Autodesk Inventor part; units mm, degrees
ref_plane "YZ Plane" through (0, 0, 0) normal (1, 0, 0) x (0, 1, 0)
ref_plane "XZ Plane" through (0, 0, 0) normal (0, 1, 0) x (-1, 0, 0)
ref_plane "XY Plane" through (0, 0, 0) normal (0, 0, 1) x (1, 0, 0)
sketch "Sketch1" plane through (0, 0, 0) normal (0, 0, 1) x (1, 0, 0)
  arc A0 (0, 0) -> (0, -180) centre (45.304, -90) ccw
  line L0 (-55.4554, -90) -> (-45.4554, -90) construction
  line L1 (0, -180) -> (0, -170) construction
  line L2 (0, 0) -> (0, -10) construction
  line L3 (0, -180) -> (10, -180) construction
  line L4 (0, 0) -> (10, 0) construction
  arc A1 (10, 0) -> (10, -180) centre (55.304, -90) ccw
  line L5 (0, 0) -> (10, 0)
  line L6 (10, -180) -> (0, -180)
  dimension "d0" = 180
  dimension "d1" = 10
  dimension "d2" = 10
  dimension "d3" = 10
  dimension "d4" = 10
  dimension "d5" = 10
extrude "Extrusion1" add sketch "Sketch1" along normal blind 10
sketch "Sketch2" plane through (0, 0, 0) normal (0, 1, 0) x (1, 0, 0)
  line L0 (-55.4554, -10) -> (0, -10)
  line L1 (0, -10) -> (0, -15)
  line L2 (0, -15) -> (0, 5)
  line L3 (0, 5) -> (6, 5)
  line L4 (0, -15) -> (6, -15)
  line L5 (6, -15) -> (18, -10)
  line L6 (6, 5) -> (18, 0)
  line L7 (18, 0) -> (18, -10)
  point P0 (0, 0)
  dimension "d8" = 5
  dimension "d9" = 20
  dimension "d10" = 6
  dimension "d11" = 13
extrude "Extrusion2" add sketch "Sketch2" along normal blind 5
sketch "Sketch3" plane through (0, -180, 0) normal (0, -1, 0) x (1, 0, 0)
  line L0 (0, -5) -> (0, 15) construction
  line L1 (0, 5) -> (-5, 5) construction
  line L2 (-5, 5) -> (0, 5) construction
  line L3 (0, 5) -> (-5, 5) construction
  line L4 (-5, 5) -> (-5, 15) construction
  line L5 (-5, 15) -> (15, 15) construction
  line L6 (15, 15) -> (15, -5) construction
  line L7 (15, -5) -> (-5, -5) construction
  line L8 (-5, -5) -> (-5, 5) construction
  line L9 (-5, 15) -> (15, 15)
  line L10 (15, -5) -> (-5, -5)
  line L11 (-5, 15) -> (-5, -5)
  line L12 (15, -5) -> (15, 15)
  point P0 (0, 0)
  dimension "d14" = 5
  dimension "d15" = 20
  dimension "d16" = 20
extrude "Extrusion3" add sketch "Sketch3" along normal blind 15
sketch "Sketch4" plane through (0, 5, 0) normal (0, 1, 0) x (1, 0, 0)
  line L0 (10, 0) -> (10, -10)
  circle A0 centre (10, -5) radius 2.5
  point P0 (0, 0)
  dimension "d19" = 5
extrude "Extrusion4" cut sketch "Sketch4" against normal blind 2
properties part number "kakidrone"
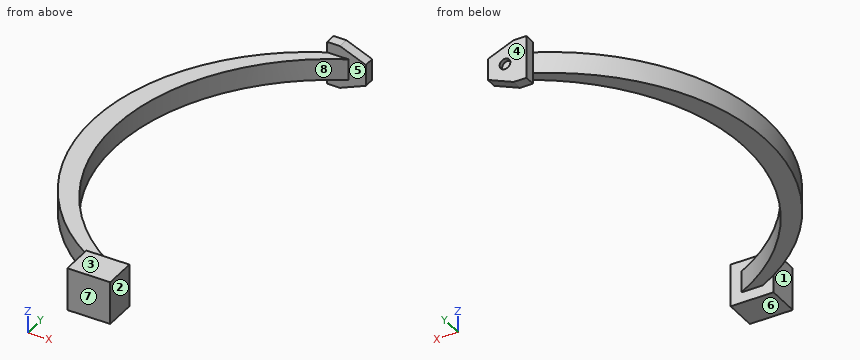
Design review of the part built by this model. Coordinates are the model's own, in mm. Face numbers are marked on the shaded views. A direction names the side the tool comes from. Give positions to 0.01 mm unless a question says otherwise; leave off trailing zeros. Loops run counter-clockwise (first coordinate to the right, second up) from the corner with the lowest first, then second, coordinate; pieces in that order, holes last. Notation, with made-up numbers: (86, 25.5) -> (94, 25.5) arc R24 ccw to (94, 61.5) -> close; hole circle Ø7 at (56.5, 74). An arc over 180 degrees is marked (long way). One line per item, written item: value.
Q1. Machinability: for the marked faces 1, 2, 3, 4 and 5, which of the approach directions +Z, -Z, +X, -X, +Y, -Y give a long, thin tool a straight path to every point of the face, cutting with its end or side? Answer none if there is none.
Numbers:
face 1: +Z, -Z, -X, -Y
face 2: +Z, -Z, +X, -Y
face 3: +Z, +X, -X, +Y, -Y
face 4: +Z, -Z, +X, -X, +Y
face 5: +X
Q2. For L1, parallel to X at y = 3.5, z = 5; L2, parallel to Y at x = 6.5, z = -1; L3, parallel to Y at x = -4.5, z = 1, list the stretches that pass through material, from the lowest coordinate up.
Numbers:
L1: x = 0 to 7.5, 12.5 to 18
L2: y = -195 to -180, 0 to 5
L3: y = -195 to -180, -177.59 to -171.09, -8.91 to -2.41
Q3. We need section C-C on y = -20.5. Give the boundary of the cut face in (x, z), and give its area (3 significant figures).
Numbers:
outline: (-27.65, 0) -> (-17.65, 0) -> (-17.65, 10) -> (-27.65, 10) -> close
area: 100 mm^2
Q4. Draft analysis for pull direction Y (two halves, no side actions). For the marked faces 6, 7 and 8, state which applies: pulls with the +Y half, pulls with the -Y half, needs draft (parallel to the pull), parting line crosses it, or undercut.
Numbers:
face 6: needs draft
face 7: pulls with the -Y half
face 8: undercut
Q5. We need section A-A on z = 12. Give the boundary of the cut face in (x, y).
Numbers:
outline: (-5, -195) -> (15, -195) -> (15, -180) -> (-5, -180) -> close; (0, 0) -> (13.2, 0) -> (13.2, 5) -> (0, 5) -> close
Q6. For pin 1 Ø4 at (x, z) = (10, 5) entering from +Y; pin 2 Ø1 at (y, z) = (-16.5, 11) entering from +X; pin 3 Ø10 at (x, z) = (-8, -0.5) entering from +Y; pin 4 Ø3 at (x, y) = (-20, -162) entering from +Z, all flat-tipped, find the tip position at first contact; note any pin that passes through.
Numbers:
pin 1: stops at y = 3
pin 2: passes through
pin 3: stops at y = -1.59
pin 4: stops at z = 10
Q7. We need section B-B on x = -29.5. Give the boundary of the cut face in (y, z).
Numbers:
outline: (-157.5, 0) -> (-144.41, 0) -> (-144.41, 10) -> (-157.5, 10) -> close; (-35.59, 0) -> (-22.5, 0) -> (-22.5, 10) -> (-35.59, 10) -> close
